Could you check a few things on this drawing? It's one solid part, dimensions in mm from its lowest x, y, z. A direction names the side the tool comes from. Round coordinates to 2 decimals unless told otherwise and drop trailing zeros. Write each loop counter-clockwise with the first axis right and the second up, starting at its lowest first coordinate (ties: lowest second). Pieces come first, ordered by that corner, then holes. Notation, with made-up numbers: (3, -6) -> (26, -6) arc R14 cw to (26, 20) -> close; hole circle Ø3 at (60, 5). An arc over 180 degrees is marked (long way). Answer in a Markdown table with one row per item.
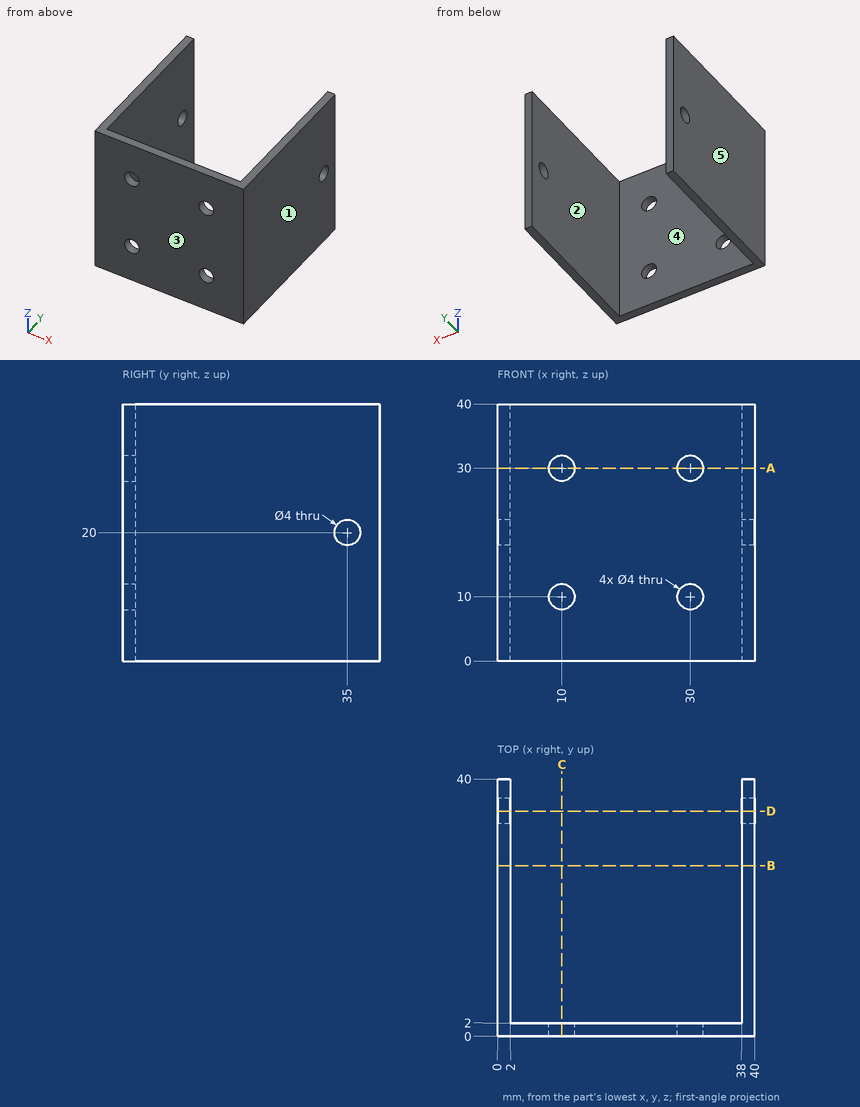
1) Imagine slicing it at D-D, the plane y = 35. Please give me the cut outline in (x, z), plus the area to 3 significant figures.
Findings:
| item | result |
|---|---|
| outline | (0, 0) -> (2, 0) -> (2, 18) -> (0, 18) -> close; (0, 22) -> (2, 22) -> (2, 40) -> (0, 40) -> close; (38, 0) -> (40, 0) -> (40, 18) -> (38, 18) -> close; (38, 22) -> (40, 22) -> (40, 40) -> (38, 40) -> close |
| area | 144 mm^2 |
2) Thinking about a two-plate mould opening in X: for the marked faces 3, 4 and 5, which applies, +X half, -X half, draft (parallel to the pull), parting line (faces both ways), or undercut?
Findings:
| item | result |
|---|---|
| face 3 | draft |
| face 4 | undercut |
| face 5 | -X half |
3) For pin 1 (2 mm diameter, centred on x = 8.5, z = 19.5, fed in from +Y); pin 2 (3 mm diameter, centred on x = 10, z = 10, fed in from +Y), each with a flat end and sliding along its axis, tell me the tip position at first contact or that it passes through.
Findings:
| item | result |
|---|---|
| pin 1 | stops at y = 2 |
| pin 2 | passes through |
4) For the marked faces 1 and 2, which set-ups out of +Z, -Z, +X, -X, +Y, -Y let a thin tool reach every point of the face, with its end or its side?
Findings:
| item | result |
|---|---|
| face 1 | +Z, -Z, +X, +Y, -Y |
| face 2 | +Z, -Z, +Y |
5) Imagine slicing it at C-C, the plane x = 10. Please give me the cut outline in (y, z).
Findings:
| item | result |
|---|---|
| outline | (0, 0) -> (2, 0) -> (2, 8) -> (0, 8) -> close; (0, 12) -> (2, 12) -> (2, 28) -> (0, 28) -> close; (0, 32) -> (2, 32) -> (2, 40) -> (0, 40) -> close |
6) Imagine slicing it at B-B, the plane y = 26.5. Please give me the cut outline in (x, z).
Findings:
| item | result |
|---|---|
| outline | (0, 0) -> (2, 0) -> (2, 40) -> (0, 40) -> close; (38, 0) -> (40, 0) -> (40, 40) -> (38, 40) -> close |
7) Please list where these lines run through material, in increasing order: line 1 (Z direction, x = 10, y = 1.4); line 2 (X direction, y = 34.5, z = 4.5).
Findings:
| item | result |
|---|---|
| line 1 | z = 0 to 8, 12 to 28, 32 to 40 |
| line 2 | x = 0 to 2, 38 to 40 |
8) Imagine slicing it at A-A, the plane z = 30. Please give me the cut outline in (x, y).
Findings:
| item | result |
|---|---|
| outline | (0, 0) -> (8, 0) -> (8, 2) -> (2, 2) -> (2, 40) -> (0, 40) -> close; (12, 0) -> (28, 0) -> (28, 2) -> (12, 2) -> close; (32, 0) -> (40, 0) -> (40, 40) -> (38, 40) -> (38, 2) -> (32, 2) -> close |
